Could you check a few things on this model? Use its own coordinates, in mm. Give positions to 0.01 mm unless a question says otherwise; leave off trailing zeros. Loops run counter-clockwise (first coordinate to the right, second up) from the corner with the lowest first, then second, coordinate; pieces in that order, holes last. Notation, with made-up numbers: M 60,-28.5 L 103,-28.5 A17 ccw 103,-11.5 Z; hole C 30,85.5 d1. An arc over 180 degrees is marked long. Return JSON: item names as keys, results as strings. Group by question number.
1. For pin 1 (1.5 mm diameter, centred on y = -0.5, z = 1.5, fed in from +X); pin 2 (1 mm diameter, centred on y = -22, z = 1.5, fed in from -X); pin 3 (1.5 mm diameter, centred on y = -9, z = 1, fed in from +X), each with a flat end and sliding along its axis, tell me the tip position at first contact or that it passes through.
2. If we section it at A-A (x = 0): Write out the boundary of the cut face in (y, z), plus the area to 3 significant figures.
3. Please list where these lines run through material, in increasing order: line 1 (Y direction, x = 0.5, z = 2.45); line 2 (X direction, y = -15.5, z = 2.55); line 3 (X direction, y = 11, z = 0.8).
4. If we section it at B-B (y = -23): Write out the boundary of the cut face in (x, z), plus the area to 3 significant figures.
5. If we section it at C-C (y = -32): Write out the boundary of the cut face in (x, z), plus the area to 3 significant figures.
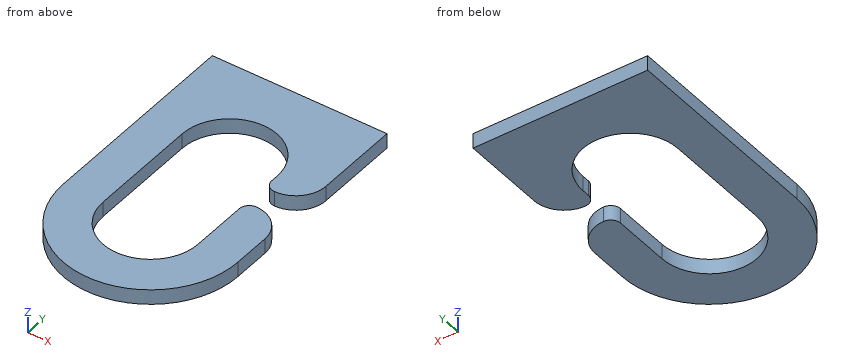
Autodesk Inventor part; units mm, degrees
ref_plane "YZ Plane" through (0, 0, 0) normal (1, 0, 0) x (0, 1, 0)
ref_plane "XZ Plane" through (0, 0, 0) normal (0, 1, 0) x (-1, 0, 0)
ref_plane "XY Plane" through (0, 0, 0) normal (0, 0, 1) x (1, 0, 0)
sketch "Sketch1" plane through (0, 0, 0) normal (0, 0, 1) x (1, 0, 0)
  line L0 (-1.5, 4) -> (1.5, 4) construction
  line L1 (1.5, 4) -> (1.5, -4) construction
  line L2 (1.5, -4) -> (-1.5, -4) construction
  line L3 (-1.5, -4) -> (-1.5, 4) construction
  line L4 (9.5, 2.5) -> (9.5, -29) construction
  line L5 (9.5, -29) -> (-9.5, -29) construction
  line L6 (-9.5, -29) -> (-9.5, 2.5)
  arc A0 (-9.5, -19.5) -> (9.5, -19.5) centre (0, -19.5) ccw
  arc A1 (-17.5, -19.5) -> (17.5, -19.5) centre (0, -19.5) ccw
  line L7 (11.5, -1) -> (20.6171, -1) construction
  line L8 (17.5, 5) -> (17.5, 22)
  line L9 (-17.5, -19.5) -> (-17.5, 22)
  line L10 (9.5, 1) -> (9.5, 2.5)
  line L11 (0, -37) -> (17.5, -37) construction
  arc A2 (11.5, -1) -> (17.5, 5) centre (11.5, 5) ccw
  arc A3 (9.5, 1) -> (11.5, -1) centre (11.5, 1) ccw
  line L12 (11.4283, -3.5) -> (20.9038, -3.5) construction
  arc A4 (17.5, -12) -> (11.5, -6) centre (11.5, -12) ccw
  arc A5 (11.5, -6) -> (9.5, -8) centre (11.5, -8) ccw
  line L13 (9.5, -8) -> (9.5, -19.5)
  line L14 (17.5, -19.5) -> (17.5, -12)
  line L15 (-17.5, 22) -> (17.5, 22)
  line L16 (-22.1996, 12) -> (26.487, 12) construction
  arc A6 (9.5, 2.5) -> (-9.5, 2.5) centre (0, 2.5) ccw
  point P0 (0, 0)
  point P1 (0, -4)
  point P2 (-1.5, 0)
  point P3 (0, -29)
  point P4 (0, 12)
  dimension "d0" = 8
  dimension "d1" = 3
  dimension "extra" = 25
  dimension "d4" = 8
  dimension "d6" = 8
  dimension "d10" = 4
  dimension "d11" = 2.5
  dimension "d12" = 3.5
  dimension "d18" = 8
  dimension "d21" = 10
  dimension "d22" = 35
extrude "Extrusion1" add sketch "Sketch1" along normal blind 3
properties part number "uhook"
Answer:
{
 "1": {"pin 1": "stops at x = 15.17", "pin 2": "stops at x = -17.39", "pin 3": "stops at x = 17.06"},
 "2": {"outline": "M -37,0 L -29,0 L -29,3 L -37,3 Z; M 12,0 L 22,0 L 22,3 L 12,3 Z", "area": "54.0 mm²"},
 "3": {"line 1": "y = -36.99 to -28.99, 11.99 to 22", "line 2": "x = -17.5 to -9.5, 9.5 to 17.5", "line 3": "x = -17.5 to -4.24, 4.24 to 17.5"},
 "4": {"outline": "M -17.15,0 L -8.83,0 L -8.83,3 L -17.15,3 Z; M 8.83,0 L 17.15,0 L 17.15,3 L 8.83,3 Z", "area": "49.9 mm²"},
 "5": {"outline": "M -12.25,0 L 12.25,0 L 12.25,3 L -12.25,3 Z", "area": "73.5 mm²"}
}
